from build123d import *

# Parameters (mm, degrees)
SKETCH_1_R           = 12.5
SKETCH_1_R_2         = 10
EXTRUDE_1_DEPTH      = 15
EXTRUDE_2_REACH      = 39.914
EXTRUDE_2_END_RADIUS = 12.5
SKETCH_2_R           = 12.5
SKETCH_2_R_2         = 10
SKETCH_3_R           = 10
CUT_EXTRUDE_1_DEPTH  = 20


with BuildPart() as part:
    # 草图1 → 凸台-拉伸1 (new, symmetric)
    with BuildSketch(Plane.XY):
        Circle(SKETCH_1_R)
        Circle(SKETCH_1_R_2, mode=Mode.SUBTRACT)
    extrude(amount=EXTRUDE_1_DEPTH, both=True)

    # 凸台-拉伸2: up to this cylinder (the profile starts outside it)
    extrude_2_end = Plane(origin=(0, 0, -12.146447), z_dir=(0, 0, -1)) * Cylinder(EXTRUDE_2_END_RADIUS, 105.828, mode=Mode.PRIVATE)
    # 草图2 → 凸台-拉伸2 (add, up to the surface)
    with BuildSketch(Plane(origin=(0, 20, 0), x_dir=(1, 0, 0), z_dir=(0, 1, 0)), mode=Mode.PRIVATE) as extrude_2_sk1:
        with Locations(Location((0, 0, 0), (0, 0, 270))):
            Circle(SKETCH_2_R)
        with Locations(Location((0, 0, 0), (0, 0, 270))):
            Circle(SKETCH_2_R_2, mode=Mode.SUBTRACT)
    extrude_2_tool1 = extrude(extrude_2_sk1.sketch, amount=-EXTRUDE_2_REACH, mode=Mode.PRIVATE) - extrude_2_end
    add(extrude_2_tool1.solids().sort_by_distance((0, 20, -12.146447))[0])

    # 草图3 → 切除-拉伸1 (cut)
    with BuildSketch(Plane(origin=(0, 20, 0), x_dir=(1, 0, 0), z_dir=(0, 1, 0))):
        with Locations(Location((0, 0, 0), (0, 0, 270))):
            Circle(SKETCH_3_R)
    extrude(amount=-CUT_EXTRUDE_1_DEPTH, mode=Mode.SUBTRACT)


solid = part.part
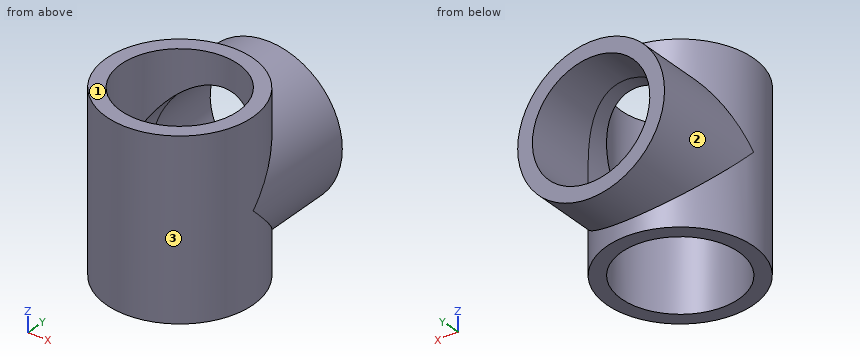
Source: CAD feature listing. Evaluate the final solid. Frame: model axes, mm. Face numbers are marked on the shaded views. A direction names the side the tool comes from. Coordinates: 2 decimals unless noted, no trailing zeros. Order: outer loops, then holes, each group sorted by start corner. A loop starts at its lowest first (then second) coordinate and runs counter-clockwise, first axis right, second up. Notation, with made-up numbers: M 42,-34 L 63,-34 A21 ccw 63,-16 Z; hole C 82,58 d9. An arc over 180 degrees is marked long. Write each question's results on one line, items separated by ' | '. Start each with the question number.
Item 1: Cut plane C-C (z = 0). Return loops of the section in (x, y).
Item 2: Cut plane B-B (y = -1.5). Return loops of the section in (x, z).
Item 3: Set-up query: the marked faces 1, 2 and 3. Return all of +Z, -Z, +X, -X, +Y, -Y with unobstructed straight access to the full face (end or side cutting, diameter ignored); none if empty.
Item 4: Cut plane A-A (x = 0). Return loops of the section in (y, z), and give its area (4 significant figures).
Item 5: Line query: probe 1 along X at (y, z) = (17.25, 0); probe 2 along Y at (x, z) = (0.25, -1.75); probe 3 along Y at (x, z) = (2.25, 13.25). Output: solid intervals per line, ascending.
Item 6: First-contact query: pin 1 Ø2 at (y, z) = (-1.5, 9.5) entering from +X; pin 2 Ø5 at (x, y) = (-2.5, 15) entering from -Z; pin 3 Ø1 at (y, z) = (8, -3) entering from -X. Flat tips, straight axial feed; report the tip coordinate or a pass-through.
Item 7: Cut plane D-D (x = 5.5). Return loops of the section in (y, z), and give its area (3 significant figures).
Checked values:
1) outline: M -12.5,0 A12.5 ccw 12.5,0 L 12.5,20 L 10,20 L 10,0 A10 cw -10,0 L -10,20 L -12.5,20 Z
2) outline: M -12.41,-15 L -9.89,-15 L -9.89,15 L -12.41,15 Z; M 9.89,-15 L 12.41,-15 L 12.41,15 L 9.89,15 Z
3) face 1: +Z, +X, -X, +Y, -Y | face 2: +Y | face 3: none
4) outline: M -12.5,-15 L -10,-15 L -10,15 L -12.5,15 Z; M 10,-15 L 12.5,-15 L 12.5,-12.5 L 20,-12.5 L 20,-10 L 10,-10 Z; M 10,10 L 20,10 L 20,12.5 L 12.5,12.5 L 12.5,15 L 10,15 Z | area: 137.5 mm2
5) probe 1: x = -12.5 to -10, 10 to 12.5 | probe 2: y = -12.5 to -10 | probe 3: y = -12.3 to -9.74, 9.74 to 12.3
6) pin 1: stops at x = 12.49 | pin 2: stops at z = -12.5 | pin 3: stops at x = -12.25
7) outline: M -11.22,-15 L -8.35,-15 L -8.35,15 L -11.22,15 Z; M 8.35,-15 L 11.22,-15 L 11.22,-11.22 L 20,-11.22 L 20,-8.35 L 8.35,-8.35 Z; M 8.35,8.35 L 20,8.35 L 20,11.22 L 11.22,11.22 L 11.22,15 L 8.35,15 Z | area: 175 mm2
